Verification items for the finished model (mm, model axes). Coordinates: 2 decimals unless noted, no trailing zeros. Order: outer loops, then holes, each group sorted by start corner. A loop starts at its lowest first (then second) coordinate and runs counter-clockwise, first axis right, second up.
Q1. Cross-section at D-D, the plane y = -10.5. Record the boundary of the cut face in (x, z), and give its area (3 significant figures).
Q2. Cross-section at A-A, the plane z = 100. Record the boundary of the cut face in (x, y), and give its area (3 significant figures).
Q3. Cross-section at B-B, the plane y = -23. Record the boundary of the cut face in (x, z).
Q4. Cross-section at C-C, the plane y = -47. Record the boundary of the cut face in (x, z).
Q5. Thickness scan on line 1 (Y direction, x = 0, z = 220); line 2 (Y direction, x = 9, z = 216); line 3 (Y direction, x = -2.5, z = 154). Record the ranges inside material, lowest first.
Q6. Depth check by flat-ended pin: P1, Ø1, axis at y = 1, z = 26.5, coming from the +X side; P2, Ø7, axis at x = -9.5, z = 54.5, coming from the +Y side; P3, Ø2, axis at y = 6, z = 108, coming from the -X side. Enter the tip coordinate at first touch or a pass-through.
from build123d import *

# Parameters (mm, degrees)
BOSS_EXTRUDE1_DEPTH      = 190
SKETCH3_R                = 1
CUT_EXTRUDE1_DEPTH       = 191.682982985
SKETCH4_W                = 3.000241119
SKETCH4_H                = 22
CUT_EXTRUDE2_DEPTH       = 191.682982985
BOSS_EXTRUDE2_DEPTH      = 14
BOSS_EXTRUDE2_DEPTH_BACK = 14
CHAMFER1_SIZE            = 10
FILLET1_R                = 2
BOSS_EXTRUDE3_DEPTH      = 12.41
SKETCH8_W                = 9.414213562
SKETCH8_H                = 53
CUT_EXTRUDE3_DEPTH       = 245.681494555
CUT_EXTRUDE4_DEPTH       = 244.772504146
CUT_EXTRUDE5_DEPTH       = 243.216914722
FILLET2_R                = 5


with BuildPart() as part:
    # Sketch2 → Boss-Extrude1 (new body)
    with BuildSketch(Plane.XY):
        Polygon((-14, -0.387014685), (-6.26397645, -0.387014685), (-3.263735331, 5.612985315), (3.263735331, 5.612985315), (6.26397645, -0.387014685), (14, -0.387014685), (14, 1.612985315), (7.5, 1.612985315), (4.499758881, 7.612985315), (-4.499758881, 7.612985315), (-7.5, 1.612985315), (-14, 1.612985315), align=None)
    extrude(amount=BOSS_EXTRUDE1_DEPTH)

    # Sketch3 → Cut-Extrude1 (cut, through all)
    with BuildSketch(Plane(origin=(0, 7.612985315, 0), x_dir=(1, 0, 0), z_dir=(0, 1, 0))):
        with Locations(Location((0, -48, 0), (0, 0, 270))):
            Circle(SKETCH3_R)
        with Locations(Location((0, -58, 0), (0, 0, 270))):
            Circle(SKETCH3_R)
        with Locations(Location((0, -68, 0), (0, 0, 270))):
            Circle(SKETCH3_R)
        with Locations(Location((0, -78, 0), (0, 0, 270))):
            Circle(SKETCH3_R)
    extrude(amount=-CUT_EXTRUDE1_DEPTH, mode=Mode.SUBTRACT)

    # Sketch4 → Cut-Extrude2 (cut, through all)
    with BuildSketch(Plane(origin=(0, 7.612985315, 0), x_dir=(1, 0, 0), z_dir=(0, 1, 0))):
        with Locations((-5.999879441, -24)):
            Rectangle(SKETCH4_W, SKETCH4_H)
        with Locations((-5.999879441, -105)):
            Rectangle(SKETCH4_W, SKETCH4_H)
        with Locations((5.999879441, -105)):
            Rectangle(SKETCH4_W, SKETCH4_H)
        with Locations((5.999879441, -24)):
            Rectangle(SKETCH4_W, SKETCH4_H)
    extrude(amount=-CUT_EXTRUDE2_DEPTH, mode=Mode.SUBTRACT)

    # Sketch5 → Boss-Extrude2 (add, two sides: drawn at the far end of the back side and taken through both)
    with BuildSketch(Plane(origin=(0, 0, 0), x_dir=(0, 0, -1), z_dir=(1, 0, 0)).offset(-BOSS_EXTRUDE2_DEPTH_BACK)):
        Polygon((-231.5, -15.387014685), (-212.5, -15.387014685), (-190, -0.387014685), (-178, 7.612985315), (-181, 7.612985315), (-190, 1.612985315), (-212.5, -13.387014685), (-231.5, -13.387014685), align=None)
    extrude(amount=BOSS_EXTRUDE2_DEPTH + BOSS_EXTRUDE2_DEPTH_BACK)

    # Chamfer1
    chamfer1_edges = [part.edges().sort_by_distance(p)[0] for p in [
        (14, -14.387014685, 231.5),
        (-14, -14.387014685, 231.5),
    ]]
    chamfer(chamfer1_edges, length=CHAMFER1_SIZE)

    # Fillet1
    fillet1_edges = [part.edges().sort_by_distance(p)[0] for p in [
        (4, -14.387014685, 231.5),
        (-4, -14.387014685, 231.5),
        (-14, -14.387014685, 221.5),
        (14, -14.387014685, 221.5),
    ]]
    fillet(fillet1_edges, radius=FILLET1_R)

    # Sketch7 → Boss-Extrude3 (add)
    with BuildSketch(Plane.XY.offset(231.5)):
        with BuildLine():
            Line((-10, -68.387014685), (10, -68.387014685))
            ThreePointArc((10, -68.387014685), (17.071067812, -65.458082497), (20, -58.387014685))
            Line((20, -58.387014685), (20, -25.387014685))
            ThreePointArc((20, -25.387014685), (17.071067812, -18.315946873), (10, -15.387014685))
            Line((10, -15.387014685), (-10, -15.387014685))
            ThreePointArc((-10, -15.387014685), (-17.071067812, -18.315946873), (-20, -25.387014685))
            Line((-20, -25.387014685), (-20, -58.387014685))
            ThreePointArc((-20, -58.387014685), (-17.071067812, -65.458082497), (-10, -68.387014685))
        make_face()
        with BuildLine():
            ThreePointArc((10.124631545, -40.717897038), (0, -20.887014685), (-10.124631545, -40.717897038))
            ThreePointArc((-10.124631545, -40.717897038), (0, -64.387014685), (10.124631545, -40.717897038))
        make_face(mode=Mode.SUBTRACT)
    extrude(amount=-BOSS_EXTRUDE3_DEPTH)

    # Sketch8 → Cut-Extrude3 (cut, through all)
    with BuildSketch(Plane(origin=(20, 0, 0), x_dir=(0, 0, -1), z_dir=(1, 0, 0))):
        with Locations((-226.792893219, -41.887014685)):
            Rectangle(SKETCH8_W, SKETCH8_H)
    extrude(amount=-CUT_EXTRUDE3_DEPTH, mode=Mode.SUBTRACT)

    # Sketch9 → Cut-Extrude4 (cut, through all)
    with BuildSketch(Plane(origin=(14, 0, 0), x_dir=(0, 0, -1), z_dir=(1, 0, 0))):
        Polygon((-190, 1.612985315), (-190, 7.612985315), (-181, 7.612985315), align=None)
    extrude(amount=-CUT_EXTRUDE4_DEPTH, mode=Mode.SUBTRACT)

    # Sketch11 → Cut-Extrude5 (cut, through all)
    with BuildSketch(Plane(origin=(0, 0, 0), x_dir=(-1, 0, 0), z_dir=(0, 0, -1))):
        Polygon((14, 7.612985315), (4.499758881, 7.612985315), (7.5, 1.612985315), (14, 1.612985315), align=None)
        Polygon((-14, 1.612985315), (-7.5, 1.612985315), (-4.499758881, 7.612985315), (-14, 7.612985315), align=None)
    extrude(amount=-CUT_EXTRUDE5_DEPTH, mode=Mode.SUBTRACT)

    # Fillet2
    fillet2_edges = [part.edges().sort_by_distance(p)[0] for p in [
        (-10.124631545, -40.717897038, 220.587893219),
        (10.124631545, -40.717897038, 220.587893219),
    ]]
    fillet(fillet2_edges, radius=FILLET2_R)


solid = part.part
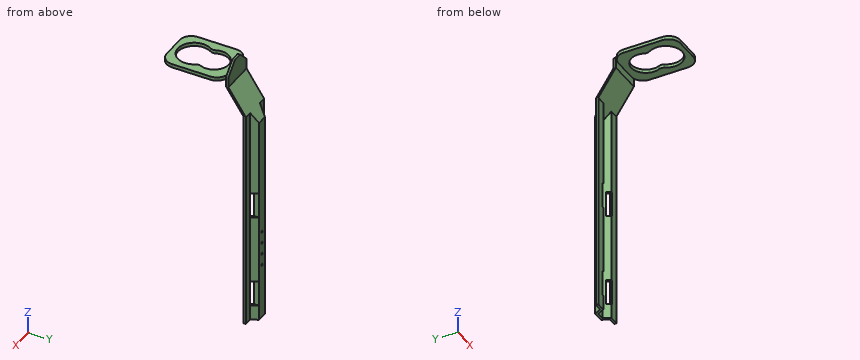
Check values:
1. outline: (-14, 205.17) - (14, 205.17) - (14, 208.17) - (-14, 208.17) - close
1. area: 84.0 mm2
2. outline: (-14, -0.39) - (-7.5, -0.39) - (-7.5, 1.61) - (-14, 1.61) - close; (-4.5, 3.14) - (-3.26, 5.61) - (3.26, 5.61) - (4.5, 3.14) - (4.5, 7.61) - (-4.5, 7.61) - close; (7.5, -0.39) - (14, -0.39) - (14, 1.61) - (7.5, 1.61) - close
2. area: 47.1 mm2
3. outline: (-19.71, 219.09) - (-6.95, 219.09) - (-6.95, 222.09) - (-19.71, 222.09) - close; (6.95, 219.09) - (19.71, 219.09) - (19.71, 222.09) - (6.95, 222.09) - close
4. outline: (-20, 219.09) - (-13.58, 219.09) - (-13.58, 222.09) - (-20, 222.09) - close; (13.58, 219.09) - (20, 219.09) - (20, 222.09) - (13.58, 222.09) - close
5. line 1: y = -68.39 to -64.39, -20.89 to -13.39
5. line 2: y = -15.39 to -13.39
5. line 3: y = 5.61 to 7.61
6. P1: stops at x = 14
6. P2: stops at y = 4.61
6. P3: stops at x = -4.5
